Source: CAD feature listing. Evaluate the final solid. Frame: model axes, mm. A direction names the side the tool comes from. Coordinates: 2 decimals unless noted, no trailing zeros. Loops run counter-clockwise (first coordinate to the right, second up) from the corner with the lowest first, then second, coordinate; pieces in that order, holes last. Notation, with made-up numbers: (-34, 63) - (4, 63) arc R21 cw to (4, 73) - close; hole circle Ø3 at (14.5, 86.5). An arc over 180 degrees is marked (long way). Use one line per item in the form item = value. Start each with the question number.
from build123d import *

# Parameters (mm, degrees)
SKETCH_1_R               = 1.6
EXTRUDE_1_DEPTH          = 10
SKETCH_3_R               = 10
EXTRUDE_2_DEPTH          = 25
CUT_EXTRUDE_1_DEPTH      = 41.311288741
CUT_EXTRUDE_1_DEPTH_BACK = 41.311288741
CUT_EXTRUDE_2_DEPTH      = 25


with BuildPart() as part:
    # ｽｹｯﾁ1 → ﾎﾞｽ - 押し出し1 (new body)
    with BuildSketch(Plane(origin=(0, 0, 0), x_dir=(1, 0, 0), z_dir=(0, 1, 0))):
        with BuildLine():
            Line((-9.797958971, -2), (-4.898979486, -26))
            ThreePointArc((-4.898979486, -26), (0, -30), (4.898979486, -26))
            Line((4.898979486, -26), (9.797958971, -2))
            ThreePointArc((9.797958971, -2), (0, 10), (-9.797958971, -2))
        make_face()
        with Locations(Location((0, -25, 0), (0, 0, 270))):
            Circle(SKETCH_1_R, mode=Mode.SUBTRACT)
    extrude(amount=EXTRUDE_1_DEPTH)

    # ｽｹｯﾁ3 → ﾎﾞｽ - 押し出し2 (add)
    with BuildSketch(Plane(origin=(0, 10, 0), x_dir=(1, 0, 0), z_dir=(0, 1, 0))):
        with Locations(Location((0, 0, 0), (0, 0, 191.536959033))):
            Circle(SKETCH_3_R)
    extrude(amount=EXTRUDE_2_DEPTH)

    # ｽｹｯﾁ2 → ｶｯﾄ - 押し出し1 (cut, two sides: drawn at the far end of the back side and taken through both)
    with BuildSketch(Plane(origin=(0, 10, 0), x_dir=(1, 0, 0), z_dir=(0, 1, 0)).offset(-CUT_EXTRUDE_1_DEPTH_BACK)):
        with BuildLine():
            Line((-1.688194302, 2.6), (-1, 2.6))
            Line((-1, 2.6), (-1, 4.6))
            Line((-1, 4.6), (1, 4.6))
            Line((1, 4.6), (1, 2.6))
            Line((1, 2.6), (1.688194302, 2.6))
            ThreePointArc((1.688194302, 2.6), (0, -3.1), (-1.688194302, 2.6))
        make_face()
    extrude(amount=CUT_EXTRUDE_1_DEPTH + CUT_EXTRUDE_1_DEPTH_BACK, mode=Mode.SUBTRACT)

    # ｽｹｯﾁ4 → ｶｯﾄ - 押し出し2 (cut)
    with BuildSketch(Plane(origin=(0, 0, 0), x_dir=(-1, 0, 0), z_dir=(0, -1, 0))):
        with BuildLine():
            Line((-4.226182617, 9.06307787), (0, 0))
            Line((0, 0), (4.226182617, 9.06307787))
            ThreePointArc((4.226182617, 9.06307787), (0, 10), (-4.226182617, 9.06307787))
        make_face()
    extrude(amount=-CUT_EXTRUDE_2_DEPTH, mode=Mode.SUBTRACT)


solid = part.part
(1) Mould query, pull axis Z, two halves, no side actions, for faces 1 (the face through (-2.7, 12.32, -5.79)), 2 (the face through (1, 30, -4)), 3 (the face through (-2, 35, 3)). Classes: +Z half, -Z half, draft (parallel to the pull), parting line (faces both ways), or undercut.
(2) Cut plane A-A, the plane z = 0. Output: boundary loops of the cut face in (x, y), plus the area to 3 significant figures.
(3) Cut plane B-B, the plane y = 31.5. Output: boundary loops of the cut face in (x, z), plus the area to 3 significant figures.
(4) Material intervals for line 1 (X direction, y = 27, z = 0); line 2 (Y direction, x = 1.25, z = 15); line 3 (Z direction, x = 0, y = 19), sorted ascending.
(5) Access query for faces 4 (the face through (0, 5, 30)), 5 (the face through (2.74, 12.32, -5.88)), 6 (the face through (0, 30, -4.6)). Directions: +Z, -Z, +X, -X, +Y, -Y. A direction counts if a zero-diameter tool reaches every point of the face in a straight line with its end or side. Return the directions, or none.
(6) Cut plane C-C, the plane x = 0. Output: boundary loops of the cut face in (y, z), plus the area to 4 significant figures.
(7) Contact query for flat-ended pins moving along their axis: pin 1 (0.6 mm diameter, centred on x = 1.5, y = 17, fed in from +Z); pin 2 (8 mm diameter, centred on x = 6, y = 28, fed in from +Z); pin 3 (4 mm diameter, centred on x = 5, y = 28, fed in from -Z). Output: stop coordinate, or through.
(8) Cut plane D-D, the plane y = 24. Output: boundary loops of the cut face in (x, z).
Recorded:
q1.face_1 = -Z half
q1.face_2 = undercut
q1.face_3 = draft
q2.outline = (-10, 0) - (-3.1, 0) - (-3.1, 35) - (-10, 35) - close; (3.1, 0) - (10, 0) - (10, 35) - (3.1, 35) - close
q2.area = 483 mm²
q3.outline = circle Ø20 at (0, 0); hole (-1.69, -2.6) - (-1, -2.6) - (-1, -4.6) - (1, -4.6) - (1, -2.6) - (1.69, -2.6) arc R3.1 ccw (long way) to start
q3.area = 281 mm²
q4.line_1 = -10 to -3.1, 3.1 to 10
q4.line_2 = 0 to 10
q4.line_3 = 3.1 to 10
q5.face_4 = +Z, +Y, -Y
q5.face_5 = -Z, -Y
q5.face_6 = +Y, -Y
q6.outline = (0, 3.1) - (35, 3.1) - (35, 10) - (10, 10) - (10, 23.4) - (0, 23.4) - close; (0, 26.6) - (10, 26.6) - (10, 30) - (0, 30) - close; (25, -10) - (35, -10) - (35, -4.6) - (25, -4.6) - close
q6.area = 463.5 mm²
q7.pin_1 = 9.93
q7.pin_2 = 9.8
q7.pin_3 = -9.54
q8.outline = (-4.23, -9.06) - (-1.21, -2.6) - (-1.69, -2.6) arc R3.1 cw (long way) to (1.69, -2.6) - (1.21, -2.6) - (4.23, -9.06) arc R10 ccw (long way) to start
